```python
from build123d import *

# Parameters (mm, degrees)
SKETCH_1_W             = 42
SKETCH_1_H             = 30
EXTRUDE_1_DEPTH        = 16
SHELL_1_T              = -2
CUT_EXTRUDE_3_REACH    = 49.381
SKETCH_4_W             = 26
SKETCH_4_H             = 2
SKETCH_5_W             = 27.6
SKETCH_5_H             = 1
CUT_EXTRUDE_4_DEPTH    = 40.8
CUT_EXTRUDE_6_REACH    = 32.364
SKETCH_8_W             = 14
SKETCH_8_H             = 2
CUT_EXTRUDE_7_REACH    = 41.962
SKETCH_9_W             = 14
SKETCH_9_H             = 2
FILLET_3_R             = 1
FILLET_4_R             = 1
FILLET_3_OF_MIRROR_1_R = 1
FILLET_4_OF_MIRROR_1_R = 1
CUT_EXTRUDE_8_REACH    = 49.381
SKETCH_10_W            = 9
SKETCH_10_H            = 4.5
CUT_EXTRUDE_9_REACH    = 41.962
SKETCH_11_W            = 11
SKETCH_11_H            = 4
FILLET_5_R             = 1
FILLET_6_R             = 0.4


# Some blends are built 0.0001 mm under size
with BuildPart() as part:
    # 草图1 → 凸台-拉伸1 (new body)
    with BuildSketch(Plane(origin=(0, 0, 0), x_dir=(1, 0, 0), z_dir=(0, 1, 0))):
        Rectangle(SKETCH_1_W, SKETCH_1_H)
    extrude(amount=EXTRUDE_1_DEPTH)

    # 抽壳1
    shell_1_openings = [part.faces().sort_by_distance(p)[0] for p in [
        (0, 16, 0),
    ]]
    offset(amount=SHELL_1_T, openings=shell_1_openings, kind=Kind.INTERSECTION)

    # 草图4 → 切除-拉伸3 (cut, up to next)
    with BuildSketch(Plane(origin=(21, 0, 0), x_dir=(0, 0, -1), z_dir=(1, 0, 0)), mode=Mode.PRIVATE) as cut_extrude_3_sk1:
        with Locations((0, 15)):
            Rectangle(SKETCH_4_W, SKETCH_4_H)
    cut_extrude_3_tool1 = extrude(cut_extrude_3_sk1.sketch, amount=-CUT_EXTRUDE_3_REACH, mode=Mode.PRIVATE) & part.part
    add(cut_extrude_3_tool1.solids().sort_by_distance((21, 15, 0))[0], mode=Mode.SUBTRACT)

    # 草图5 → 切除-拉伸4 (cut)
    with BuildSketch(Plane(origin=(21, 0, 0), x_dir=(0, 0, -1), z_dir=(1, 0, 0))):
        with Locations((0, 14.5)):
            Rectangle(SKETCH_5_W, SKETCH_5_H)
    extrude(amount=-CUT_EXTRUDE_4_DEPTH, mode=Mode.SUBTRACT)

    # 草图8 → 切除-拉伸6 (cut, up to next)
    with BuildSketch(Plane.XZ, mode=Mode.PRIVATE) as cut_extrude_6_sk1:
        with Locations((0, -12)):
            Rectangle(SKETCH_8_W, SKETCH_8_H)
    cut_extrude_6_tool1 = extrude(cut_extrude_6_sk1.sketch, amount=-CUT_EXTRUDE_6_REACH, mode=Mode.PRIVATE) & part.part
    cut_extrude_6 = cut_extrude_6_tool1.solids().sort_by_distance((0, 0, -12))[0]
    add(cut_extrude_6, mode=Mode.SUBTRACT)

    # 草图9 → 切除-拉伸7 (cut, up to next)
    with BuildSketch(Plane(origin=(0, 0, -15), x_dir=(-1, 0, 0), z_dir=(0, 0, -1)), mode=Mode.PRIVATE) as cut_extrude_7_sk1:
        with Locations((0, 3)):
            Rectangle(SKETCH_9_W, SKETCH_9_H)
    cut_extrude_7_tool1 = extrude(cut_extrude_7_sk1.sketch, amount=-CUT_EXTRUDE_7_REACH, mode=Mode.PRIVATE) & part.part
    cut_extrude_7 = cut_extrude_7_tool1.solids().sort_by_distance((0, 3, -15))[0]
    add(cut_extrude_7, mode=Mode.SUBTRACT)

    # 圆角3
    # the kernel refuses this fillet: 1 mm, written as the material it adds along each edge
    with BuildSketch(Plane(origin=(-7, 4, -15), x_dir=(0, -1, 0), z_dir=(0, 0, 1)), Plane(origin=(-7, 2, -15), x_dir=(1, 0, 0), z_dir=(0, 0, 1)), Plane(origin=(7, 2, -15), x_dir=(0, 1, 0), z_dir=(0, 0, 1))) as fillet_3_piece_1:
        with BuildLine():
            CenterArc((FILLET_3_R, FILLET_3_R), FILLET_3_R, 180, 90)
            Line((0, FILLET_3_R), (0, 0))
            Line((0, 0), (FILLET_3_R, 0))
        make_face()
    extrude(amount=2)
    with BuildSketch(Plane(origin=(7, 4, -15), x_dir=(0, -1, 0), z_dir=(0, 0, 1))) as fillet_3_piece_2:
        with BuildLine():
            CenterArc((FILLET_3_R, -FILLET_3_R), FILLET_3_R, 90, 90)
            Line((0, -FILLET_3_R), (0, 0))
            Line((0, 0), (FILLET_3_R, 0))
        make_face()
    extrude(amount=2)

    # 圆角4
    fillet_4_edges = [part.edges().sort_by_distance(p)[0] for p in [
        (-7, 1, -13),
        (-7, 1, -11),
        (7, 1, -13),
        (7, 1, -11),
    ]]
    fillet(fillet_4_edges, radius=FILLET_4_R - 0.0001)  # a hair under: the kernel refuses the full size

    # 镜向1: 切除-拉伸6, 切除-拉伸7 across plane
    add(cut_extrude_6.mirror(Plane.XY), mode=Mode.SUBTRACT)
    add(cut_extrude_7.mirror(Plane.XY), mode=Mode.SUBTRACT)

    # 圆角3 of 镜向1
    # the kernel refuses this fillet: 1 mm, written as the material it adds along each edge
    with BuildSketch(Plane(origin=(-7, 4, 15), x_dir=(1, 0, 0), z_dir=(0, 0, -1)), Plane(origin=(-7, 2, 15), x_dir=(0, 1, 0), z_dir=(0, 0, -1)), Plane(origin=(7, 2, 15), x_dir=(-1, 0, 0), z_dir=(0, 0, -1))) as fillet_3_of_mirror_1_piece_1:
        with BuildLine():
            CenterArc((FILLET_3_OF_MIRROR_1_R, FILLET_3_OF_MIRROR_1_R), FILLET_3_OF_MIRROR_1_R, 180, 90)
            Line((0, FILLET_3_OF_MIRROR_1_R), (0, 0))
            Line((0, 0), (FILLET_3_OF_MIRROR_1_R, 0))
        make_face()
    extrude(amount=2)
    with BuildSketch(Plane(origin=(7, 4, 15), x_dir=(-1, 0, 0), z_dir=(0, 0, -1))) as fillet_3_of_mirror_1_piece_2:
        with BuildLine():
            CenterArc((FILLET_3_OF_MIRROR_1_R, -FILLET_3_OF_MIRROR_1_R), FILLET_3_OF_MIRROR_1_R, 90, 90)
            Line((0, -FILLET_3_OF_MIRROR_1_R), (0, 0))
            Line((0, 0), (FILLET_3_OF_MIRROR_1_R, 0))
        make_face()
    extrude(amount=2)

    # 圆角4 of 镜向1
    fillet_4_of_mirror_1_edges = [part.edges().sort_by_distance(p)[0] for p in [
        (-7, 1, 13),
        (-7, 1, 11),
        (7, 1, 13),
        (7, 1, 11),
    ]]
    fillet(fillet_4_of_mirror_1_edges, radius=FILLET_4_OF_MIRROR_1_R - 0.0001)  # a hair under: the kernel refuses the full size

    # 草图10 → 切除-拉伸8 (cut, up to next)
    with BuildSketch(Plane.ZY.offset(21), mode=Mode.PRIVATE) as cut_extrude_8_sk1:
        with Locations((-8.5, 9.25)):
            Rectangle(SKETCH_10_W, SKETCH_10_H)
    cut_extrude_8_tool1 = extrude(cut_extrude_8_sk1.sketch, amount=-CUT_EXTRUDE_8_REACH, mode=Mode.PRIVATE) & part.part
    add(cut_extrude_8_tool1.solids().sort_by_distance((-21, 9.25, -8.5))[0], mode=Mode.SUBTRACT)

    # 草图11 → 切除-拉伸9 (cut, up to next)
    with BuildSketch(Plane(origin=(0, 0, -15), x_dir=(-1, 0, 0), z_dir=(0, 0, -1)), mode=Mode.PRIVATE) as cut_extrude_9_sk1:
        with Locations((-10.5, 12)):
            Rectangle(SKETCH_11_W, SKETCH_11_H)
    cut_extrude_9_tool1 = extrude(cut_extrude_9_sk1.sketch, amount=-CUT_EXTRUDE_9_REACH, mode=Mode.PRIVATE) & part.part
    add(cut_extrude_9_tool1.solids().sort_by_distance((10.5, 12, -15))[0], mode=Mode.SUBTRACT)

    # 圆角5
    fillet_5_edges = [part.edges().sort_by_distance(p)[0] for p in [
        (16, 14, -14.4),
        (16, 10, -14),
        (5, 14, -14.4),
        (5, 10, -14),
    ]]
    fillet(fillet_5_edges, radius=FILLET_5_R)

    # 圆角6
    fillet_6_edges = [part.edges().sort_by_distance(p)[0] for p in [
        (-20, 7, -4),
        (-20, 11.5, -4),
        (-20, 11.5, -13),
        (-20, 7, -13),
    ]]
    fillet(fillet_6_edges, radius=FILLET_6_R)


solid = part.part
```
Geometry check sheet. Reference: the model listing, model coordinates, mm. A direction names the side the tool comes from. Coordinates: 2 decimals unless noted, no trailing zeros. Order: outer loops, then holes, each group sorted by start corner. A loop starts at its lowest first (then second) coordinate and runs counter-clockwise, first axis right, second up.
Item 1: Section check A-A (y = 3). Enter the section's corners in (x, z).
Item 2: Scan lines: line 1 along Z through (x, y) = (0, 1); line 2 along X through (y, z) = (6.5, -3.75); line 3 along Z through (x, y) = (5, 9). Record each from-to range of solid material in increasing order.
Item 3: Depth check by flat-ended pin: pin 1 (10 mm diameter, centred on x = 13.5, z = 2, fed in from +Y); pin 2 (0.8 mm diameter, centred on y = 15.5, z = 1, fed in from +X). Enter the tip coordinate at first touch or a pass-through.
Item 4: Mould release check, pull along X, two halves, no side actions. Record for faces 5 (the flat face through (-21, 8, 0)), 6 (the flat face through (0, 0, 0)), 7 (the flat face through (11, 10, -14)): released by +X, released by -X, zero draft, split by the parting line, or undercut.
Item 5: Section check B-B (x = 0). Enter the section's corners in (y, z), plus the area to 3 significant figures.
Item 6: Section check C-C (y = 5.5). Enter the section's corners in (x, z).
Item 7: Tool access check on faces 1 (the cylindrical face through (15.699, 10.285, -13.986)), 2 (the flat face through (0.9, 14.5, 13.8)), 3 (the cylindrical face through (-6.715, 1.014, 12.699)), 4 (the cylindrical face through (-7, 3, 14)). Record the directions out of +Z, -Z, +X, -X, +Y, -Y that give a thin tool (end or side, any length) a straight path to the whole face; none if there is none.
Item 8: Section check D-D (x = 10). Enter the section's corners in (y, z).
Check sheet entries:
1. outline: (-21, -15) - (-7, -15) - (-7, -13) - (-19, -13) - (-19, 13) - (-7, 13) - (-7, 15) - (-21, 15) - close; (7, -15) - (21, -15) - (21, 15) - (7, 15) - (7, 13) - (19, 13) - (19, -13) - (7, -13) - close
2. line 1: z = -15 to -13, -11 to 11, 13 to 15
2. line 2: x = -21 to -19, 19 to 21
2. line 3: z = -15 to -13, 13 to 15
3. pin 1: stops at y = 2
3. pin 2: stops at x = -19
4. face 5: released by -X
4. face 6: zero draft
4. face 7: undercut
5. outline: (0, -15) - (2, -15) - (2, -13) - (0, -13) - close; (0, -11) - (2, -11) - (2, 11) - (0, 11) - close; (0, 13) - (2, 13) - (2, 15) - (0, 15) - close; (4, -15) - (16, -15) - (16, -13) - (15, -13) - (15, -13.8) - (14, -13.8) - (14, -13) - (4, -13) - close; (4, 13) - (14, 13) - (14, 13.8) - (15, 13.8) - (15, 13) - (16, 13) - (16, 15) - (4, 15) - close
5. area: 98.4 mm2
6. outline: (-21, -15) - (21, -15) - (21, 15) - (-21, 15) - close; hole (-19, -13) - (19, -13) - (19, 13) - (-19, 13) - close
7. face 1: -Z
7. face 2: +X
7. face 3: +Y, -Y
7. face 4: +Z, -Z
8. outline: (0, -15) - (10, -15) - (10, -13) - (2, -13) - (2, 13) - (14, 13) - (14, 13.8) - (15, 13.8) - (15, 13) - (16, 13) - (16, 15) - (0, 15) - close; (14, -15) - (16, -15) - (16, -13) - (15, -13) - (15, -13.8) - (14, -13.8) - close
